from build123d import *

# Parameters (mm, degrees)
F2_W           = 75
F2_H           = 2
F4_R           = 3
F6_DEPTH       = 2
F9_D           = 5.5
F9_DEPTH       = 18
F9_TIP         = 1.6523667023
F9_ON_F7_D     = 5.5
F9_ON_F7_DEPTH = 18
F9_ON_F7_TIP   = 1.6523667023


with BuildPart() as f3:
    # F3: sweep along a path in F0
    with BuildLine(Plane.XZ) as f3_path:
        Line((-80, 0), (0, 0))
        Line((0, 0), (0, 80))
        Line((0, 80), (-40, 80))
    # F2 (on line) → F3 (sweep)
    with BuildSketch(Plane.YZ.offset(-80)):
        Rectangle(F2_W, F2_H)
    sweep(path=f3_path.line, transition=Transition.RIGHT)

    # F4
    f4_edges = [f3.edges().sort_by_distance(p)[0] for p in [
        (-1, 0, 1),
        (-1, 0, 79),
        (1, 0, -1),
        (1, 0, 81),
    ]]
    fillet(f4_edges, radius=F4_R)

    # F5 (on face) → F6 (cut, through all)
    with BuildSketch(Plane.XY.offset(81)):
        with BuildLine():
            ThreePointArc((-40, -25), (-22.3223304703, -17.6776695297), (-15, 0))
            ThreePointArc((-15, 0), (-22.3223304703, 17.6776695297), (-40, 25))
            Line((-40, 25), (-40, -25))
        make_face()
    extrude(amount=-F6_DEPTH, mode=Mode.SUBTRACT)

    # F9
    with Locations(Plane.XY.offset(81)):
        with Locations((-35, 28.5), (-10, 0), (-35, -28.5)):
            Hole(F9_D / 2, depth=F9_DEPTH)
            with Locations((0, 0, -(F9_DEPTH + F9_TIP / 2))):  # 118° drill point
                Cone(0, F9_D / 2, F9_TIP, mode=Mode.SUBTRACT)

    # F9 on F7
    with Locations(Plane(origin=(0, 0, -1), x_dir=(1, 0, 0), z_dir=(0, 0, -1))):
        with Locations((-30, 20), (-30, -20), (-70, -20), (-70, 20)):
            Hole(F9_ON_F7_D / 2, depth=F9_ON_F7_DEPTH)
            with Locations((0, 0, -(F9_ON_F7_DEPTH + F9_ON_F7_TIP / 2))):  # 118° drill point
                Cone(0, F9_ON_F7_D / 2, F9_ON_F7_TIP, mode=Mode.SUBTRACT)


solid = f3.part
Design review of the part built by this model. Coordinates are the model's own, in mm. A direction names the side the tool comes from. Coordinates: 2 decimals unless noted, no trailing zeros. Loops run counter-clockwise (first coordinate to the right, second up) from the corner with the lowest first, then second, coordinate; pieces in that order, holes last. Notation, with made-up numbers: M 12,-21 L 36,-21 A36 ccw 36,14 Z; hole C 66,84.5 d3. An arc over 180 degrees is marked long. Answer as CSV lines item,"result".
Item 1: Add section D-D on x = -35. State the section outline as (y, z) points.
Answer list:
outline,"M -37.5,-1 L 37.5,-1 L 37.5,1 L -37.5,1 Z; M -37.5,79 L -31.25,79 L -31.25,81 L -37.5,81 Z; M -25.75,79 L -24.49,79 L -24.49,81 L -25.75,81 Z; M 24.49,79 L 25.75,79 L 25.75,81 L 24.49,81 Z; M 31.25,79 L 37.5,79 L 37.5,81 L 31.25,81 Z"
Item 2: For P1, Ø1, axis at y = -34, z = 80.5, coming from the -X side; P2, Ø4, axis at y = -27, z = 8, coming from the -X side; P3, Ø5, axis at x = -10, y = 0, coming from the +Z side, all flat-tipped, find the tip position at first contact; note any pin that passes through.
Answer list:
P1,"x = -40"
P2,"x = -1"
P3,"z = 1"
Item 3: For probe 1 along Y at (x, z) = (-30, 0); probe 2 along Y at (x, z) = (-10, 79.8); probe 3 along X at (y, z) = (-20, -0.3), list the stretches that pass through material, from the lowest coordinate up.
Answer list:
probe 1,"-37.5 to -22.75, -17.25 to 17.25, 22.75 to 37.5"
probe 2,"-37.5 to -2.75, 2.75 to 37.5"
probe 3,"-80 to -72.75, -67.25 to -32.75, -27.25 to -0.07"
Item 4: Add section A-A on x = -70. State the section outline as (y, z) points, plus the area to 3 significant figures.
Answer list:
outline,"M -37.5,-1 L -22.75,-1 L -22.75,1 L -37.5,1 Z; M -17.25,-1 L 17.25,-1 L 17.25,1 L -17.25,1 Z; M 22.75,-1 L 37.5,-1 L 37.5,1 L 22.75,1 Z"
area,"128 mm²"
Item 5: The part is to be moulded in two halves that separate along Y. For faces 1 (the face through (0, 37.5, 31)), 2 (the face through (1, -1, 41)), 3 (the face through (0, -37.5, 31)), 4 (the face through (-12.54, -1.05, 79.99)), say which applies: pulls with the +Y half, pulls with the -Y half, needs draft (parallel to the pull), parting line crosses it, or undercut.
Answer list:
face 1,"pulls with the +Y half"
face 2,"needs draft"
face 3,"pulls with the -Y half"
face 4,"undercut"
Item 6: Machinability: for faces 5 (the face through (-1, 1, 41)), 6 (the face through (0.1, -0.52, -0.14)), 7 (the face through (-32.253, -28.379, 79.986)), which of the approach directions +Z, -Z, +X, -X, +Y, -Y give a long, thin tool a straight path to every point of the face, cutting with its end or side? Answer none if there is none.
Answer list:
face 5,"-X, +Y, -Y"
face 6,"-Z, +X, +Y, -Y"
face 7,"+Z"
Item 7: Add section C-C on y = -28.5. State the section outline as (x, z) points, plus the area to 3 significant figures.
Answer list:
outline,"M -80,-1 L -2,-1 A3 ccw 1,2 L 1,78 A3 ccw -2,81 L -32.25,81 L -32.25,79 L -4,79 A3 cw -1,76 L -1,4 A3 cw -4,1 L -80,1 Z; M -40,79 L -37.75,79 L -37.75,81 L -40,81 Z"
area,"389 mm²"
Item 8: Add section B-B on y = -20. State the section outline as (x, z) points.
Answer list:
outline,"M -80,-1 L -72.75,-1 L -72.75,1 L -80,1 Z; M -67.25,-1 L -32.75,-1 L -32.75,1 L -67.25,1 Z; M -27.25,-1 L -2,-1 A3 ccw 1,2 L 1,78 A3 ccw -2,81 L -25,81 L -25,79 L -4,79 A3 cw -1,76 L -1,4 A3 cw -4,1 L -27.25,1 Z"
